from build123d import *

# Parameters (mm, degrees)
F1_DEPTH      = 5
F3_DEPTH      = 10
F5_DEPTH      = 25
F6_R          = 1.5
F7_DEPTH      = 69.4
F8_R          = 6.7597979746
F9_R          = 5
F10_R         = 5
F11_T1_DEPTH  = 45.7
F11_T3_DEPTH  = 45.7
F12_T1_DEPTH  = 54.4
F12_T3_DEPTH  = 30
F12_T5_DEPTH  = 38
F12_S9_W      = 5
F12_S9_H      = 5
F12_T10_DEPTH = 5
F12_S15_W     = 5
F12_S15_H     = 5
F12_T16_DEPTH = 5
F12_S21_W     = 5
F12_S21_H     = 5
F12_T22_DEPTH = 5
F12_S27_W     = 5
F12_S27_H     = 5
F12_T28_DEPTH = 5
F12_T32_ANGLE = 90
F12_T34_ANGLE = 90


# Not quite as in the source:
# - a fillet or chamfer that OpenCascade refuses, or shapes differently, is made with other operations: its cross-section is extruded or revolved along the edge and cut away or added


with BuildPart() as f1:
    # F0 (on Front) → F1 (new body)
    with BuildSketch(Plane.XZ):
        with BuildLine():
            Line((32.2, -24), (32.2, 24))
            Line((32.2, 24), (6.5, 24))
            Line((6.5, 24), (6.5, 10.8))
            Line((6.5, 10.8), (8.4, 10.8))
            Line((8.4, 10.8), (8.4, 14.8))
            ThreePointArc((8.4, 14.8), (14.9, 21.3), (21.4, 14.8))
            Line((21.4, 14.8), (21.4, 10.8))
            Line((21.4, 10.8), (24.4, 10.8))
            Line((24.4, 10.8), (24.4, -10.8))
            Line((24.4, -10.8), (21.4, -10.8))
            Line((21.4, -10.8), (21.4, -14.8))
            ThreePointArc((21.4, -14.8), (14.9, -21.3), (8.4, -14.8))
            Line((8.4, -14.8), (8.4, -10.8))
            Line((8.4, -10.8), (-8.4, -10.8))
            Line((-8.4, -10.8), (-8.4, -14.8))
            ThreePointArc((-8.4, -14.8), (-14.9, -21.3), (-21.4, -14.8))
            Line((-21.4, -14.8), (-21.4, -10.8))
            Line((-21.4, -10.8), (-24.4, -10.8))
            Line((-24.4, -10.8), (-24.4, 10.8))
            Line((-24.4, 10.8), (-21.4, 10.8))
            Line((-21.4, 10.8), (-21.4, 14.8))
            ThreePointArc((-21.4, 14.8), (-14.9, 21.3), (-8.4, 14.8))
            Line((-8.4, 14.8), (-8.4, 10.8))
            Line((-8.4, 10.8), (-6.5, 10.8))
            Line((-6.5, 10.8), (-6.5, 24))
            Line((-6.5, 24), (-32.2, 24))
            Line((-32.2, 24), (-32.2, -24))
            Line((-32.2, -24), (32.2, -24))
        make_face()
    extrude(amount=F1_DEPTH)

    # F2 (on face) → F3 (join)
    with BuildSketch(Plane(origin=(0, 0, 0), x_dir=(-1, 0, 0), z_dir=(0, 1, 0))):
        with BuildLine():
            Line((24.4, 10.8), (24.4, -10.8))
            Line((24.4, -10.8), (21.4, -10.8))
            Line((21.4, -10.8), (21.4, -14.8))
            ThreePointArc((21.4, -14.8), (14.9, -21.3), (8.4, -14.8))
            Line((8.4, -14.8), (8.4, -10.8))
            Line((8.4, -10.8), (-8.4, -10.8))
            Line((-8.4, -10.8), (-8.4, -14.8))
            ThreePointArc((-8.4, -14.8), (-14.9, -21.3), (-21.4, -14.8))
            Line((-21.4, -14.8), (-21.4, -10.8))
            Line((-21.4, -10.8), (-24.4, -10.8))
            Line((-24.4, -10.8), (-24.4, 10.8))
            Line((-24.4, 10.8), (-21.4, 10.8))
            Line((-21.4, 10.8), (-21.4, 14.8))
            ThreePointArc((-21.4, 14.8), (-14.9, 21.3), (-8.4, 14.8))
            Line((-8.4, 14.8), (-8.4, 10.8))
            Line((-8.4, 10.8), (-6.5, 10.8))
            Line((-6.5, 10.8), (-6.5, 24))
            Line((-6.5, 24), (-32.2, 24))
            Line((-32.2, 24), (-32.2, -24))
            Line((-32.2, -24), (32.2, -24))
            Line((32.2, -24), (32.2, 24))
            Line((32.2, 24), (6.5, 24))
            Line((6.5, 24), (6.5, 10.8))
            Line((6.5, 10.8), (8.4, 10.8))
            Line((8.4, 10.8), (8.4, 14.8))
            ThreePointArc((8.4, 14.8), (14.9, 21.3), (21.4, 14.8))
            Line((21.4, 14.8), (21.4, 10.8))
            Line((21.4, 10.8), (24.4, 10.8))
        make_face()
        with BuildLine():
            Line((21.4, -14.8), (21.4, -10.8))
            Line((21.4, -10.8), (8.4, -10.8))
            Line((8.4, -10.8), (8.4, -14.8))
            ThreePointArc((8.4, -14.8), (14.9, -21.3), (21.4, -14.8))
        make_face()
        with BuildLine():
            Line((-8.4, -14.8), (-8.4, -10.8))
            Line((-8.4, -10.8), (-21.4, -10.8))
            Line((-21.4, -10.8), (-21.4, -14.8))
            ThreePointArc((-21.4, -14.8), (-14.9, -21.3), (-8.4, -14.8))
        make_face()
        with BuildLine():
            Line((8.4, 10.8), (21.4, 10.8))
            Line((21.4, 10.8), (21.4, 14.8))
            ThreePointArc((21.4, 14.8), (14.9, 21.3), (8.4, 14.8))
            Line((8.4, 14.8), (8.4, 10.8))
        make_face()
        with BuildLine():
            Line((-21.4, 10.8), (-8.4, 10.8))
            Line((-8.4, 10.8), (-8.4, 14.8))
            ThreePointArc((-8.4, 14.8), (-14.9, 21.3), (-21.4, 14.8))
            Line((-21.4, 14.8), (-21.4, 10.8))
        make_face()
    extrude(amount=F3_DEPTH)

    # F4 (on face) → F5 (join)
    with BuildSketch(Plane(origin=(0, 10, 0), x_dir=(-1, 0, 0), z_dir=(0, 1, 0))):
        Polygon((32.2, -24), (32.2, 24), (6.5, 24), (6.5, 10.8), (24.4, 10.8), (24.4, -10.8), (-24.4, -10.8), (-24.4, 10.8), (-6.5, 10.8), (-6.5, 24), (-32.2, 24), (-32.2, -24), align=None)
        Polygon((6.5, 10.8), (6.5, 24), (-6.5, 24), (-6.5, 10.8), (-24.4, 10.8), (-24.4, -10.8), (24.4, -10.8), (24.4, 10.8), align=None)
        with BuildLine():
            ThreePointArc((5.5288725662, 5.5), (16.8680666762, 9.6842239514), (24.1, 0))
            ThreePointArc((24.1, 0), (16.8680666762, -9.6842239514), (5.5288725662, -5.5))
            Line((5.5288725662, -5.5), (0, -5.5))
            Line((0, -5.5), (-5.5288725662, -5.5))
            ThreePointArc((-5.5288725662, -5.5), (-24.1, 0), (-5.5288725662, 5.5))
            Line((-5.5288725662, 5.5), (0, 5.5))
            Line((0, 5.5), (5.5288725662, 5.5))
        make_face(mode=Mode.SUBTRACT)
    extrude(amount=F5_DEPTH)

    # F6 (on face) → F7 (cut)
    with BuildSketch(Plane(origin=(-32.2, 0, 0), x_dir=(0, -1, 0), z_dir=(-1, 0, 0))):
        with Locations((-13.5, 16.806252715)):
            Circle(F6_R)
    extrude(amount=-F7_DEPTH, mode=Mode.SUBTRACT)

    # F8
    f8_edges = [f1.edges().sort_by_distance(p)[0] for p in [
        (0, 35, 24),
    ]]
    fillet(f8_edges, radius=F8_R)

    # F9
    f9_edges = [f1.edges().sort_by_distance(p)[0] for p in [
        (32.2, 33.020101, 22.020101),
        (32.2, 35, -3.379899),
    ]]
    fillet(f9_edges, radius=F9_R)

    # F10
    f10_edges = [f1.edges().sort_by_distance(p)[0] for p in [
        (-32.2, 35, -3.379899),
    ]]
    fillet(f10_edges, radius=F10_R)

    # F11: fillet of radius 5 on 2 edges, made by hand

    # F11_s2 → F11_t1 (cut)
    with BuildSketch(Plane.YZ.offset(-39.7)):
        with BuildLine():
            ThreePointArc((-5, 19), (-3.5355339059, 22.5355339059), (0, 24))
            Line((0, 24), (-5, 24))
            Line((-5, 24), (-5, 19))
        make_face()
    extrude(amount=F11_T1_DEPTH, mode=Mode.SUBTRACT)

    # F11_s4 → F11_t3 (cut)
    with BuildSketch(Plane.YZ.offset(-6)):
        with BuildLine():
            ThreePointArc((-5, 19), (-3.5355339059, 22.5355339059), (0, 24))
            Line((0, 24), (-5, 24))
            Line((-5, 24), (-5, 19))
        make_face()
    extrude(amount=F11_T3_DEPTH, mode=Mode.SUBTRACT)

    # F12: fillet of radius 5 on 8 edges, made by hand

    # F12_s2 → F12_t1 (cut)
    with BuildSketch(Plane.YZ.offset(-27.2)):
        with BuildLine():
            ThreePointArc((30, -24), (33.5355339059, -22.5355339059), (35, -19))
            Line((35, -19), (35, -24))
            Line((35, -24), (30, -24))
        make_face()
        with BuildLine():
            ThreePointArc((0, -24), (-3.5355339059, -22.5355339059), (-5, -19))
            Line((-5, -19), (-5, -24))
            Line((-5, -24), (0, -24))
        make_face()
    extrude(amount=F12_T1_DEPTH, mode=Mode.SUBTRACT)

    # F12_s4 → F12_t3 (cut)
    with BuildSketch(Plane.XZ.offset(-30)):
        with BuildLine():
            ThreePointArc((-27.2, -24), (-30.7355339059, -22.5355339059), (-32.2, -19))
            Line((-32.2, -19), (-32.2, -24))
            Line((-32.2, -24), (-27.2, -24))
        make_face()
        with BuildLine():
            ThreePointArc((27.2, -24), (30.7355339059, -22.5355339059), (32.2, -19))
            Line((32.2, -19), (32.2, -24))
            Line((32.2, -24), (27.2, -24))
        make_face()
    extrude(amount=F12_T3_DEPTH, mode=Mode.SUBTRACT)

    # F12_s6 → F12_t5 (cut)
    with BuildSketch(Plane.XY.offset(-19)):
        with BuildLine():
            ThreePointArc((-32.2, 0), (-30.7355339059, -3.5355339059), (-27.2, -5))
            Line((-27.2, -5), (-32.2, -5))
            Line((-32.2, -5), (-32.2, 0))
        make_face()
        with BuildLine():
            ThreePointArc((32.2, 0), (30.7355339059, -3.5355339059), (27.2, -5))
            Line((27.2, -5), (32.2, -5))
            Line((32.2, -5), (32.2, 0))
        make_face()
    extrude(amount=F12_T5_DEPTH, mode=Mode.SUBTRACT)


with BuildPart() as f12_tool8:
    # F12_s9 → F12_t10 (new body)
    with BuildSketch(Plane.YZ.offset(27.2)):
        with Locations((-2.5, 21.5)):
            Rectangle(F12_S9_W, F12_S9_H)
    extrude(amount=F12_T10_DEPTH)

    # F12_s11 → F12_t12 (revolve, cut)
    with BuildSketch(Plane(origin=(27.2, 0, 19), x_dir=(0, 0.7071067812, -0.7071067812), z_dir=(0, -0.7071067812, -0.7071067812))):
        with BuildLine():
            ThreePointArc((0, -5), (5, 0), (0, 5))
            Line((0, 5), (0, -5))
        make_face()
    revolve(axis=Axis((27.2, 0, 19), (1, 0, 0)), mode=Mode.SUBTRACT)


with BuildPart() as f1_1:
    add(f1.part)

    # F12_t7: cut F12_tool8
    add(f12_tool8.part, mode=Mode.SUBTRACT)


with BuildPart() as f12_tool14:
    # F12_s15 → F12_t16 (new body)
    with BuildSketch(Plane.YZ.offset(-27.2)):
        with Locations((-2.5, 21.5)):
            Rectangle(F12_S15_W, F12_S15_H)
    extrude(amount=-F12_T16_DEPTH)

    # F12_s17 → F12_t18 (revolve, cut)
    with BuildSketch(Plane(origin=(-27.2, 0, 19), x_dir=(0, 0.7071067812, -0.7071067812), z_dir=(0, 0.7071067812, 0.7071067812))):
        with BuildLine():
            ThreePointArc((0, -5), (5, 0), (0, 5))
            Line((0, 5), (0, -5))
        make_face()
    revolve(axis=Axis((-27.2, 0, 19), (-1, 0, 0)), mode=Mode.SUBTRACT)


with BuildPart() as f1_2:
    add(f1_1.part)

    # F12_t13: cut F12_tool14
    add(f12_tool14.part, mode=Mode.SUBTRACT)


with BuildPart() as f12_tool20:
    # F12_s21 → F12_t22 (new body)
    with BuildSketch(Plane.XY.offset(-19)):
        with Locations((-29.7, -2.5)):
            Rectangle(F12_S21_W, F12_S21_H)
    extrude(amount=-F12_T22_DEPTH)

    # F12_s23 → F12_t24 (revolve, cut)
    with BuildSketch(Plane(origin=(-27.2, 0, -19), x_dir=(0.7071067812, 0.7071067812, 0), z_dir=(-0.7071067812, 0.7071067812, 0))):
        with BuildLine():
            ThreePointArc((0, -5), (5, 0), (0, 5))
            Line((0, 5), (0, -5))
        make_face()
    revolve(axis=Axis((-27.2, 0, -19), (0, 0, -1)), mode=Mode.SUBTRACT)


with BuildPart() as f1_3:
    add(f1_2.part)

    # F12_t19: cut F12_tool20
    add(f12_tool20.part, mode=Mode.SUBTRACT)


with BuildPart() as f12_tool26:
    # F12_s27 → F12_t28 (new body)
    with BuildSketch(Plane.XY.offset(-19)):
        with Locations((29.7, -2.5)):
            Rectangle(F12_S27_W, F12_S27_H)
    extrude(amount=-F12_T28_DEPTH)

    # F12_s29 → F12_t30 (revolve, cut)
    with BuildSketch(Plane(origin=(27.2, 0, -19), x_dir=(-0.7071067812, 0.7071067812, 0), z_dir=(-0.7071067812, -0.7071067812, 0))):
        with BuildLine():
            ThreePointArc((0, -5), (5, 0), (0, 5))
            Line((0, 5), (0, -5))
        make_face()
    revolve(axis=Axis((27.2, 0, -19), (0, 0, -1)), mode=Mode.SUBTRACT)


with BuildPart() as f1_4:
    add(f1_3.part)

    # F12_t25: cut F12_tool26
    add(f12_tool26.part, mode=Mode.SUBTRACT)

    # F12_s31 → F12_t32 (revolve, cut)
    with BuildSketch(Plane.YZ.offset(-27.2)):
        with BuildLine():
            ThreePointArc((30, -24), (33.5355339059, -22.5355339059), (35, -19))
            Line((35, -19), (35, -24))
            Line((35, -24), (30, -24))
        make_face()
    revolve(axis=Axis((-27.2, 30, -24), (0, 0, 1)), revolution_arc=F12_T32_ANGLE, mode=Mode.SUBTRACT)

    # F12_s33 → F12_t34 (revolve, cut)
    with BuildSketch(Plane.XZ.offset(-30)):
        with BuildLine():
            ThreePointArc((27.2, -24), (30.7355339059, -22.5355339059), (32.2, -19))
            Line((32.2, -19), (32.2, -24))
            Line((32.2, -24), (27.2, -24))
        make_face()
    revolve(axis=Axis((27.2, 30, -24), (0, 0, 1)), revolution_arc=F12_T34_ANGLE, mode=Mode.SUBTRACT)


solid = f1_4.part
CAD build for the part. Positions are in the model's coordinates, mm. A direction names the side the tool comes from. Give positions to 0.01 mm unless a question says otherwise; leave off trailing zeros. Loops run counter-clockwise (first coordinate to the right, second up) from the corner with the lowest first, then second, coordinate; pieces in that order, holes last. Notation, with made-up numbers: M 21.25,9 L 60.25,9 A21 cw 60.25,48 Z; hole C 18.25,81 d5. An arc over 180 degrees is marked long. Answer in a Markdown table with one row per item. Add a question column.
Item 1: Tool access for faces 5 (the face through (-15, 0, -16)), 6 (the face through (24.093, 22.325, -0.363)): list every direction of +Z, -Z, +X, -X, +Y, -Y with a clear straight run to the whole face (end or side of a thin tool).
Item 2: Band-saw the part on A-A on y = 13.5. Give the cut face in (x, z).
Item 3: Drop flat-ended pins along their axis: P1, Ø11.5, axis at x = 16, z = -14.5, coming from the -Y side; P2, Ø4.5, axis at y = -2.5, z = -12, coming from the -X side; P3, Ø4.5, axis at y = -3.5, z = 12.5, coming from the +X side; P4, Ø3, axis at y = -2.5, z = 13.5, coming from the +X side. Give the stop position or say it passes through.
Item 4: Mould opens along Y. For faces 1 (the face through (-0.451, 14.606, 17.82)), 2 (the face through (0, 33, -23)), 3 (the face through (25, -5, 0)), 4 (the face through (0, 4, -10.8)) say: +Y half, -Y half, draft (parallel to the pull), parting line (faces both ways), or undercut.
Item 5: Band-saw the part on D-D on z = 14. Give the cut face in (x, y).
Item 6: Band-saw the part on C-C on y = 18.5. Give the cut face in (x, z), then the cut area to 3 significant figures.
Item 7: Probe probe 1 along X at (y, z) = (6, 16); probe 2 along X at (y, z) = (1.5, 10.5); probe 3 along Z at (x, y) = (14, 20). List the from-to ranges inside material, lowest first.
Item 8: Band-saw the part on B-B on x = 15.5. Give the cut face in (y, z).
Reply:
| question | item | result |
|---|---|---|
| 1 | face 5 | -Y |
| 1 | face 6 | +Y, -Y |
| 2 | outline | M -32.2,-19 A5 ccw -27.2,-24 L 27.2,-24 A5 ccw 32.2,-19 L 32.2,15.31 L -32.2,15.31 Z; M -32.2,18.31 L 32.2,18.31 L 32.2,19 A5 ccw 27.2,24 L -27.2,24 A5 ccw -32.2,19 Z; hole M -5.53,-5.5 L 5.53,-5.5 A10.1 ccw long 5.53,5.5 L -5.53,5.5 A10.1 ccw long Z |
| 3 | P1 | stops at y = -5 |
| 3 | P2 | stops at x = -32.19 |
| 3 | P3 | stops at x = 32.04 |
| 3 | P4 | stops at x = 32.1 |
| 4 | face 1 | undercut |
| 4 | face 2 | +Y half |
| 4 | face 3 | -Y half |
| 4 | face 4 | draft |
| 5 | outline | M -32.2,0 A5 ccw -27.2,-5 L -21.4,-5 L -21.4,0 L -8.4,0 L -8.4,-5 L -6.5,-5 L -6.5,10 L 6.5,10 L 6.5,-5 L 8.4,-5 L 8.4,0 L 21.4,0 L 21.4,-5 L 27.2,-5 A5 ccw 32.2,0 L 32.2,30 A5 ccw 27.2,35 L -27.2,35 A5 ccw -32.2,30 Z |
| 6 | outline | M -32.2,-19 A5 ccw -27.2,-24 L 27.2,-24 A5 ccw 32.2,-19 L 32.2,19 A5 ccw 27.2,24 L -27.2,24 A5 ccw -32.2,19 Z; hole M -5.53,-5.5 L 5.53,-5.5 A10.1 ccw long 5.53,5.5 L -5.53,5.5 A10.1 ccw long Z |
| 6 | area | 2,330 mm^2 |
| 7 | probe 1 | x = -32.2 to -6.5, 6.5 to 32.2 |
| 7 | probe 2 | x = -32.2 to -24.4, 24.4 to 32.2 |
| 7 | probe 3 | z = -24 to -10.1, 10.1 to 24 |
| 8 | outline | M -4.45,-21.27 A5 ccw 0,-24 L 30,-24 A5 ccw 35,-19 L 35,-9.99 L 10,-9.99 L 10,-10.8 L 0,-10.8 L 0,-21.27 Z; M -4.45,21.27 L 0,21.27 L 0,10.8 L 10,10.8 L 10,9.99 L 35,9.99 L 35,17.24 A6.76 ccw 28.24,24 L 0,24 A5 ccw Z; hole C 13.5,16.81 d3 |
